Verification items for the finished model (mm, model axes). A direction names the side the tool comes from. Give positions to 0.01 mm unless a question says otherwise; leave off trailing zeros. Write each loop counter-clockwise with the first axis right and the second up, starting at its lowest first coordinate (ties: lowest second). Pieces come first, ordered by that corner, then holes. Notation, with made-up numbers: (39.25, -30.75) - (61.25, -30.75) arc R18 ccw to (61.25, 4.25) - close; hole circle Ø11 at (40, -36.75). An arc over 180 degrees is marked (long way). Put each result on its own line as item: value.
from build123d import *

# Parameters (mm, degrees)
F1_DEPTH = 63.5
F2_DEPTH = 25.4
F3_DEPTH = 7.9375
F5_R     = 6.35
F6_R     = 12.7
F7_DEPTH = 50.8


with BuildPart() as f1:
    # F0 (on Front) → F1 (new body, symmetric)
    with BuildSketch(Plane.XZ):
        Polygon((22.225, 9.525), (-41.275, 9.525), (-41.275, -9.525), (41.275, -9.525), (41.275, 9.525), align=None)
    extrude(amount=F1_DEPTH, both=True)

    # F0 (on Front) → F2 (join, symmetric)
    with BuildSketch(Plane.XZ):
        with BuildLine():
            Line((22.225, 27.0002), (22.225, 9.525))
            Line((22.225, 9.525), (41.275, 9.525))
            Line((41.275, 9.525), (41.275, 27.0002))
            ThreePointArc((41.275, 27.0002), (45.9246798487, 38.2255201513), (57.15, 42.8752))
            Line((57.15, 42.8752), (57.15, 61.9252))
            add(Edge.make_bspline(
                [(52.9911566186, 61.6766999204), (54.4399345917, 61.780290683), (55.8288716771, 61.8622040359), (57.15, 61.9252)],
                knots=[0.6317574931, 0.6317574931, 0.6317574931, 0.6317574931, 0.6639097579, 0.6639097579, 0.6639097579, 0.6639097579], degree=3))
            ThreePointArc((52.9911566186, 61.6766999204), (31.0252681344, 50.1789404738), (22.225, 27.0002))
        make_face()
        with BuildLine():
            Line((72.6181762576, 61.9252), (57.15, 61.9252))
            Line((57.15, 61.9252), (57.15, 42.8752))
            Line((57.15, 42.8752), (85.725, 42.8752))
            Line((85.725, 42.8752), (85.725, 61.9252))
            add(Edge.make_bspline(
                [(72.6181762576, 61.9252), (77.3737433111, 61.7384817546), (81.2709365488, 61.5258076735), (85.725, 61.9252)],
                knots=[0.8210339091, 0.8210339091, 0.8210339091, 0.8210339091, 1, 1, 1, 1], degree=3))
        make_face()
    extrude(amount=F2_DEPTH, both=True)

    # F0 (on Front) → F3 (join, symmetric)
    with BuildSketch(Plane.XZ):
        with BuildLine():
            add(Edge.make_bspline(
                [(-41.275, 9.525), (-27.0460967422, 49.236584083), (24.5242244587, 59.6412526224), (52.9911566186, 61.6766999204)],
                knots=[0, 0, 0, 0, 0.6317574931, 0.6317574931, 0.6317574931, 0.6317574931], degree=3))
            Line((-41.275, 9.525), (22.225, 9.525))
            Line((22.225, 9.525), (22.225, 27.0002))
            ThreePointArc((22.225, 27.0002), (31.0252681344, 50.1789404738), (52.9911566186, 61.6766999204))
        make_face()
    extrude(amount=F3_DEPTH, both=True)

    # F0 (on Front) → F4 (revolve)
    with BuildSketch(Plane.XZ):
        Polygon((133.35, 66.675), (85.725, 66.675), (85.725, 61.9252), (85.725, 42.8752), (85.725, 38.1), (133.35, 38.1), align=None)
    revolve(axis=Axis((85.725, 0, 52.3875), (0, 0, -1)))

    # F5
    f5_edges = [f1.edges().sort_by_distance(p)[0] for p in [
        (41.275, -63.5, 0),
        (-41.275, -63.5, 0),
        (-41.275, 63.5, 0),
        (41.275, 63.5, 0),
    ]]
    fillet(f5_edges, radius=F5_R)

    # F6 (on face) → F7 (cut)
    with BuildSketch(Plane.XZ.offset(7.9375)):
        with Locations((0, 25.5429092795)):
            Circle(F6_R)
    extrude(amount=-F7_DEPTH, mode=Mode.SUBTRACT)


solid = f1.part
Q1. Section check C-C, the plane y = -52. Record the cut outline in (x, z) (3 decimals).
Answers follow:
outline: (-41.275, -9.525) - (41.275, -9.525) - (41.275, 9.525) - (-41.275, 9.525) - close
Q2. Section check B-B, the plane x = 94.5. Record the cut outline in (y, z) (3 decimals).
Answers follow:
outline: (-46.81, 38.1) - (46.81, 38.1) - (46.81, 66.675) - (-46.81, 66.675) - close
Q3. Scan lines: line 1 along Z through (x, y) = (75, -23.5) (3 decimals); line 2 along Z through (x, y) = (0, 1) (3 decimals); line 3 along Z through (x, y) = (-33, -56.5) (3 decimals). Record each from-to range of solid material in increasing order.
Answers follow:
line 1: z = 38.1 to 66.675
line 2: z = -9.525 to 12.843, 38.243 to 49.505
line 3: z = -9.525 to 9.525
Q4. Section check A-A, the plane y = 18. Record the cut outline in (x, z) (3 decimals), plus the area to 3 significant figures.
Answers follow:
outline: (-41.275, -9.525) - (41.275, -9.525) - (41.275, 27) arc R15.875 cw to (45.801, 38.1) - (129.817, 38.1) - (129.817, 66.675) - (41.633, 66.675) - (41.633, 58.289) arc R34.925 ccw to (22.225, 27) - (22.225, 9.525) - (-41.275, 9.525) - close
area: 4,870 mm2
Q5. Go/stop test with flat-tipped pins: pin 1 Ø8 at (x, y) = (-22.5, 5.5) entering from +Z; pin 2 Ø4 at (y, z) = (45, 2) entering from +X (3 decimals); pin 3 Ø5 at (y, z) = (17, 16.5) entering from -X (3 decimals). Record where each tip stops, or that it passes through.
Answers follow:
pin 1: stops at z = 39.06
pin 2: stops at x = 41.275
pin 3: stops at x = 22.225
Q6. Set-up check for faces 1 (the face through (-41.275, -1, 0)), 2 (the face through (-39.464, -61.59, -0.133)), 3 (the face through (22.225, -17, 18)), 4 (the face through (28.8, 16.5, 47.4)), 5 (the face through (41.275, -1, 4)): record each of +Z, -Z, +X, -X, +Y, -Y from which the full face is reachable in a straight line by a thin tool's end or side.
Answers follow:
face 1: +Z, -Z, -X, +Y, -Y
face 2: +Z, -Z, -X, -Y
face 3: +Z, -X, -Y
face 4: +Z, -X, +Y
face 5: -Z, +X, +Y, -Y
